Geometry: final body of the model. Coordinates: model frame, mm. Face numbers are marked on the shaded views. Give positions to 0.01 mm unless a question says otherwise; leave off trailing zeros. Order: outer loops, then holes, each group sorted by start corner. A loop starts at its lowest first (then second) coordinate and runs counter-clockwise, first axis right, second up. Notation, with made-up numbers: (-26, 30) -> (0, 30) arc R20 ccw to (0, 62) -> close; hole circle Ø7 at (-17.5, 74). An arc over 180 degrees is marked (long way). One line per question, with ' | ' between items.
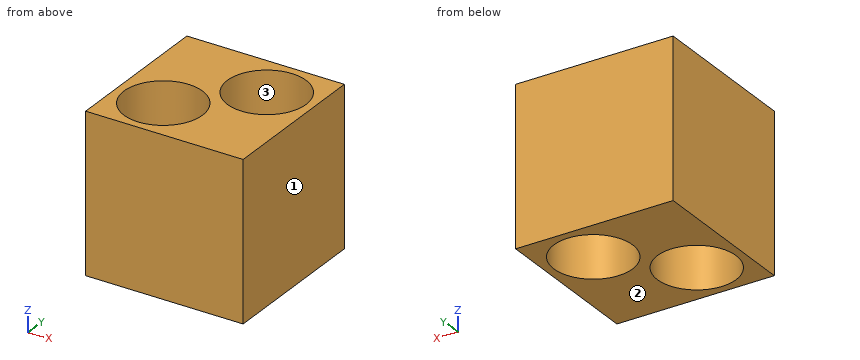
from build123d import *

# Parameters (mm, degrees)
SKETCH1_W           = 10
SKETCH1_H           = 10
BOSS_EXTRUDE1_DEPTH = 10
SKETCH2_R           = 2.5
CUT_EXTRUDE1_DEPTH  = 18.320508076


with BuildPart() as part:
    # Sketch1 → Boss-Extrude1 (new body)
    with BuildSketch(Plane.XY):
        with Locations((5, 5)):
            Rectangle(SKETCH1_W, SKETCH1_H)
    extrude(amount=BOSS_EXTRUDE1_DEPTH)

    # Sketch2 → Cut-Extrude1 (cut, through all)
    with BuildSketch(Plane.XY):
        with Locations((3, 3)):
            Circle(SKETCH2_R)
        with Locations((7, 7)):
            Circle(SKETCH2_R)
    extrude(amount=CUT_EXTRUDE1_DEPTH, mode=Mode.SUBTRACT)


solid = part.part
1) Pull-direction query (X, two-part tool) for the marked faces 1, 2 and 3; classes: +X half, -X half, draft (parallel to the pull), parting line (faces both ways), or undercut.
Check result:
face 1: +X half | face 2: draft | face 3: undercut
2) Section C-C on z = 6. Return loops of the section in (x, y).
Check result:
outline: (0, 0) -> (10, 0) -> (10, 10) -> (0, 10) -> close; hole circle Ø5 at (3, 3); hole circle Ø5 at (7, 7)
3) Section A-A on x = 9. Return loops of the section in (y, z), plus the area to 3 significant figures.
Check result:
outline: (0, 0) -> (5.5, 0) -> (5.5, 10) -> (0, 10) -> close; (8.5, 0) -> (10, 0) -> (10, 10) -> (8.5, 10) -> close | area: 70.0 mm^2
4) Material intervals for probe 1 along X at (y, z) = (7, 6.5); probe 2 along Y at (x, z) = (5, 2), sorted ascending. Write a range as from..to.
Check result:
probe 1: x = 0..4.5, 9.5..10 | probe 2: y = 0..1.5, 4.5..5.5, 8.5..10
5) Section B-B on y = 7. Return loops of the section in (x, z), plus the area to 3 significant figures.
Check result:
outline: (0, 0) -> (4.5, 0) -> (4.5, 10) -> (0, 10) -> close; (9.5, 0) -> (10, 0) -> (10, 10) -> (9.5, 10) -> close | area: 50.0 mm^2
